The figure shows three views and two pictorial views of one solid part (mm, origin at its lowest corner). Answer the questions. A direction names the side the tool comes from. Round coordinates to 2 decimals unless told otherwise and drop trailing zeros. Loops run counter-clockwise (first coordinate to the right, second up) from the corner with the lowest first, then second, coordinate; pieces in that order, holes last. Notation, with made-up numbers: (-8, 15.5) -> (27, 15.5) arc R21 ccw to (27, 51.5) -> close; hole circle Ø8 at (40, 1). An arc over 180 degrees is marked (long way). Use a Markdown table: item, result. Add a question column.
Q1. Section B-B on x = 58 is taken. Give the vertices of the cut face in (y, z).
Q2. Which of the six approach directions +Z, -Z, +X, -X, +Y, -Y give full straight-line access (tool end or side, diameter ignored) to the marked faces 4, 5 and 6?
Q3. Section C-C on z = 1.6 is taken. Give the vertices of the cut face in (x, y).
Q4. Section D-D on x = 22.5 is taken. Give the vertices of the cut face in (y, z), then the cut area to 3 significant figures.
Q5. For a pull along X with two mould halves and no side action, classify the marked faces 1, 2 and 3 as released by +X, released by -X, zero draft, split by the parting line, or undercut.
Q6. Consider line 1 (X direction, y = 5.2, z = 2.4); line 2 (X direction, y = 5.4, z = 4.05); line 3 (Z direction, x = 56.5, y = 3.9). Determine where each line is inside the solid, lowest interval first.
Q7. Given pin 1 Ø3 at (x, y) = (58, 3) entering from -Z; pin 2 Ø0.9 at (y, z) = (2, 4) entering from +X; pin 3 Ø3 at (x, y) = (56.5, 3) entering from +Z, each flat-ended and moving along its own axis, determine where each tip first touches the part or whether it passes through.
Q8. Section A-A on y = 3 is taken. Give the vertices of the cut face in (x, z).
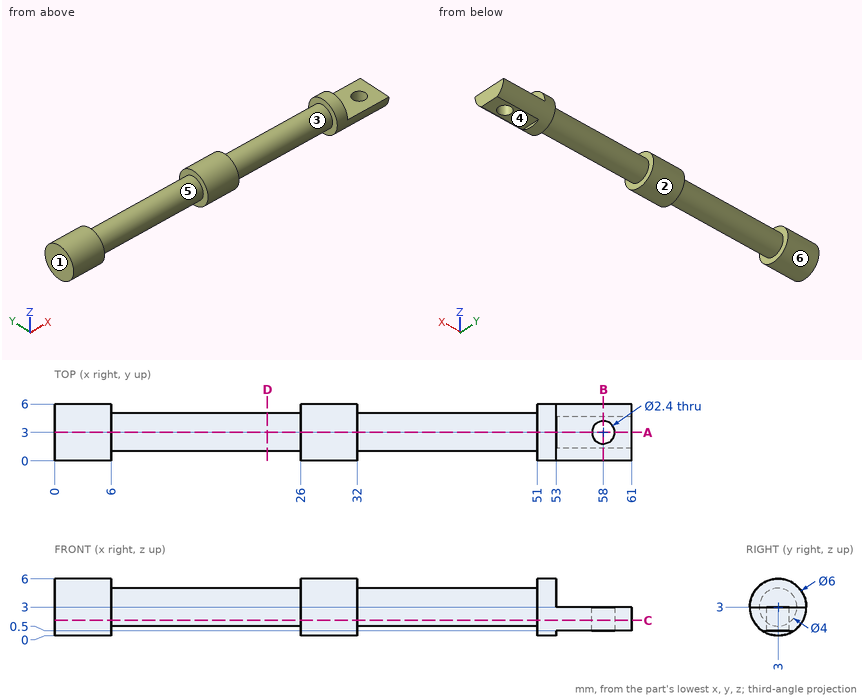
Checked values:
| question | item | result |
|---|---|---|
| 1 | outline | (0, 3) arc R3 ccw to (1.34, 0.5) -> (1.8, 0.5) -> (1.8, 3) -> close; (4.2, 0.5) -> (4.66, 0.5) arc R3 ccw to (6, 3) -> (4.2, 3) -> close |
| 2 | face 4 | -Z, +X, +Y, -Y |
| 2 | face 5 | none |
| 2 | face 6 | +X, -X |
| 3 | outline | (0, 0.35) -> (6, 0.35) -> (6, 1.57) -> (26, 1.57) -> (26, 0.35) -> (32, 0.35) -> (32, 1.57) -> (51, 1.57) -> (51, 0.35) -> (61, 0.35) -> (61, 5.65) -> (51, 5.65) -> (51, 4.43) -> (32, 4.43) -> (32, 5.65) -> (26, 5.65) -> (26, 4.43) -> (6, 4.43) -> (6, 5.65) -> (0, 5.65) -> close; hole circle Ø2.4 at (58, 3) |
| 4 | outline | circle Ø4 at (3, 3) |
| 4 | area | 12.6 mm2 |
| 5 | face 1 | released by -X |
| 5 | face 2 | zero draft |
| 5 | face 3 | undercut |
| 6 | line 1 | x = 0 to 6, 26 to 32, 51 to 61 |
| 6 | line 2 | x = 0 to 6, 26 to 32, 51 to 53 |
| 6 | line 3 | z = 0.5 to 3 |
| 7 | pin 1 | stops at z = 0.5 |
| 7 | pin 2 | stops at x = 53 |
| 7 | pin 3 | stops at z = 3 |
| 8 | outline | (0, 0) -> (6, 0) -> (6, 1) -> (26, 1) -> (26, 0) -> (32, 0) -> (32, 1) -> (51, 1) -> (51, 0) -> (53, 0) -> (53, 0.5) -> (56.8, 0.5) -> (56.8, 3) -> (53, 3) -> (53, 6) -> (51, 6) -> (51, 5) -> (32, 5) -> (32, 6) -> (26, 6) -> (26, 5) -> (6, 5) -> (6, 6) -> (0, 6) -> close; (59.2, 0.5) -> (61, 0.5) -> (61, 3) -> (59.2, 3) -> close |
